Input: dimensioned drawing with shaded views. Units: mm. Origin: part minimum x, y, z. A direction names the side the tool comes from. Coordinates: 2 decimals unless noted, no trailing zeros. Loops run counter-clockwise (first coordinate to the right, second up) from the corner with the lowest first, then second, coordinate; pieces in that order, holes last.
Item 1: Pull-direction query (X, two-part tool) for the marked faces 3, 4 and 5; classes: +X half, -X half, draft (parallel to the pull), parting line (faces both ways), or undercut.
Item 2: Line query: probe 1 along Z at (x, y) = (39.5, 117.5); probe 2 along Y at (x, z) = (61.5, 27); probe 3 along Y at (x, z) = (68.5, 28.5). Output: solid intervals per line, ascending.
Item 3: Pin query (flat end, axial travel): pin 1 Ø4 at (x, y) = (55, 57) entering from +Z; pin 2 Ø12 at (y, z) = (30, 28) entering from -X; pin 3 Ø2 at (x, z) = (70.5, 28) entering from +Y; pin 4 Ø1.4 at (x, z) = (25.5, 26.5) entering from -Y. Return the tip coordinate at first contact, or that it passes through.
Item 4: Section query A-A, the plane x = 58. Return the cut outline in (y, z), then the cut area to 3 significant figures.
Item 5: Section query B-B, the plane y = 57.5. Return the cut outline in (x, z).
Item 6: Reachability of the marked faces 1 and 2 from +Z, -Z, +X, -X, +Y, -Y: full face, straight path, thin tool, end or side. Return the list, or none.
Item 7: Section query C-C, the plane y = 130.5. Return the cut outline in (x, z).
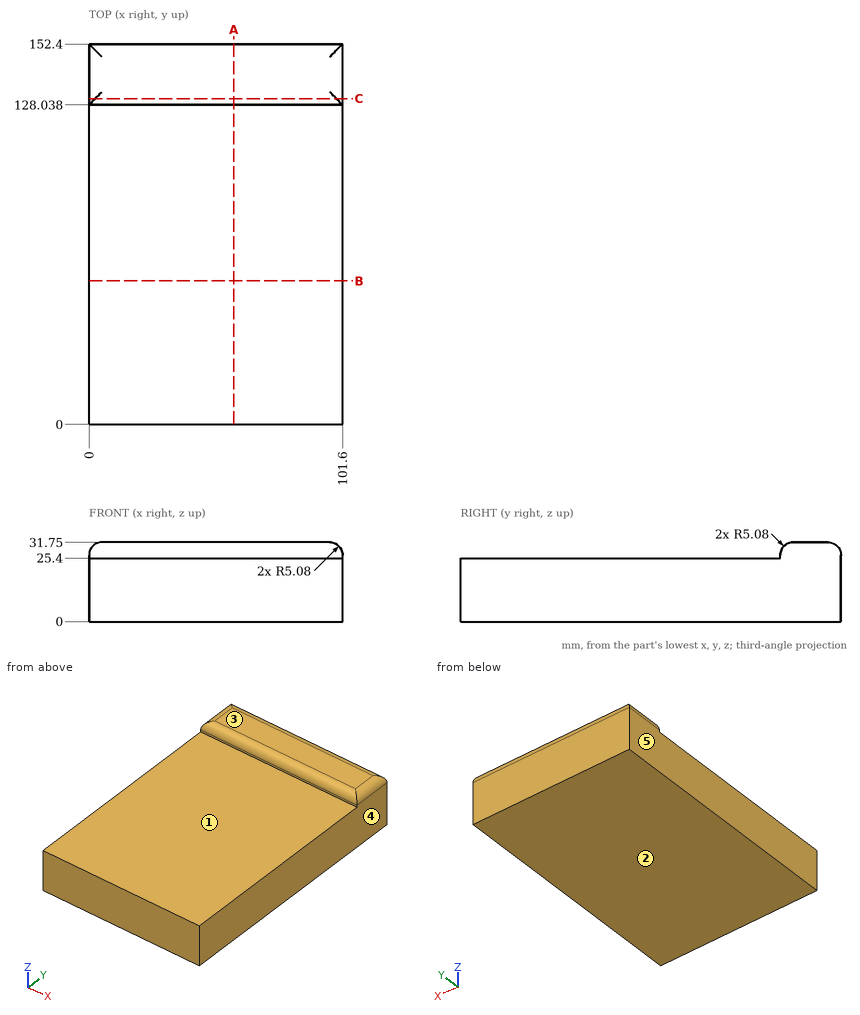
Verdict:
1. face 3: draft
1. face 4: +X half
1. face 5: -X half
2. probe 1: z = 0 to 25.4
2. probe 2: y = 128.05 to 152.39
2. probe 3: y = 128.38 to 152.06
3. pin 1: stops at z = 25.4
3. pin 2: stops at x = 0
3. pin 3: stops at y = 152.39
3. pin 4: stops at y = 128.04
4. outline: (0, 0) - (152.4, 0) - (152.4, 26.67) arc R5.08 ccw to (147.32, 31.75) - (133.12, 31.75) arc R5.08 ccw to (128.04, 26.67) - (128.04, 25.4) - (0, 25.4) - close
4. area: 4,010 mm2
5. outline: (0, 0) - (101.6, 0) - (101.6, 25.4) - (0, 25.4) - close
6. face 1: +Z, +X, -X, -Y
6. face 2: -Z, +X, -X, +Y, -Y
7. outline: (0, 0) - (101.6, 0) - (101.6, 26.67) arc R5.08 ccw to (99.14, 31.02) - (2.46, 31.02) arc R5.08 ccw to (0, 26.67) - close
